```python
from build123d import *

# Parameters (mm, degrees)
F1_DEPTH = 3.175


with BuildPart() as f1:
    # F0 (on Front) → F1 (new body)
    with BuildSketch(Plane.XZ):
        Polygon((-109.02407, -38.0746), (-136.525, -38.0746), (-136.525, 0.0254), (-86.268388, 0.0254), (-38.200188, 0.0254), (136.525, 0.0254), (136.525, -38.0746), (0, -38.0746), (-16.379747, -38.0746), (-17.745636, -41.2496), (139.7, -41.2496), (139.7, 0.0254), (177.8, 0.0254), (177.8, 3.229479), (117.504079, 63.5254), (-117.504079, 63.5254), (-177.829079, 3.2004), (-177.8, 0.0254), (-139.7, 0.0254), (-139.7, -41.2496), (-61.467241, -41.2496), (-63.375022, -38.0746), (-86.524069, -38.0746), align=None)
        Polygon((-141.752446, 3.415089), (-173.407102, 3.132249), (-152.280724, 24.258627), (-116.353083, 60.186267), (-115.853459, 60.18446), (-76.571651, 60.042381), (-33.768375, 59.887564), (117.197821, 59.34153), (170.335695, 6.203656), (0, 4.681674), (-33.768375, 4.379947), (-51.768549, 4.219112), (-51.998988, 3.506442), (-52.306652, 4.214304), (-92.559852, 3.854634), (-131.528538, 3.506442), (-138.940506, 3.440214), align=None, mode=Mode.SUBTRACT)
    extrude(amount=F1_DEPTH)


solid = f1.part
```
Can you work these out from the model? Positions are in its coordinate system, mm. Give positions to 0.01 mm unless a question says otherwise; leave off trailing zeros. Write each loop counter-clockwise with the first axis right and the second up, starting at its lowest first coordinate (ties: lowest second). Pieces come first, ordered by that corner, then holes. Notation, with made-up numbers: (-16.5, -40) -> (14.5, -40) arc R3 cw to (14.5, -35) -> close; hole circle Ø9 at (-15, 83). An arc over 180 degrees is marked (long way). Write item = value, one per line.
(1) Thinking about a two-plate mould opening in X: for faces 1 (the face through (12, 0, 4)), 2 (the face through (143.395, -1.565, 33.145)), 3 (the face through (-147.24, -1.57, 33.79)), 4 (the face through (148.07, -1.57, 32.96)), which applies, released by +X, released by -X, zero draft, split by the parting line, or undercut?
Worked out:
face_1 = zero draft
face_2 = undercut
face_3 = released by -X
face_4 = released by +X
(2) Suppose I cut it at B-B on x = 4.5. Write out the boundary of the cut face in (y, z) (3 decimals).
Worked out:
outline = (-3.175, -41.25) -> (0, -41.25) -> (0, -38.075) -> (-3.175, -38.075) -> close; (-3.175, 0.025) -> (0, 0.025) -> (0, 4.722) -> (-3.175, 4.722) -> close; (-3.175, 59.749) -> (0, 59.749) -> (0, 63.525) -> (-3.175, 63.525) -> close
(3) Suppose I cut it at D-D on x = 81.5. Write out the boundary of the cut face in (y, z) (3 decimals), then the cut area to 3 significant figures.
Worked out:
outline = (-3.175, -41.25) -> (0, -41.25) -> (0, -38.075) -> (-3.175, -38.075) -> close; (-3.175, 0.025) -> (0, 0.025) -> (0, 5.41) -> (-3.175, 5.41) -> close; (-3.175, 59.471) -> (0, 59.471) -> (0, 63.525) -> (-3.175, 63.525) -> close
area = 40.1 mm^2
(4) Suppose I cut it at C-C on x = -56.5. Write out the boundary of the cut face in (y, z) (3 decimals).
Worked out:
outline = (-3.175, 0.025) -> (0, 0.025) -> (0, 4.177) -> (-3.175, 4.177) -> close; (-3.175, 59.97) -> (0, 59.97) -> (0, 63.525) -> (-3.175, 63.525) -> close
(5) I need wall thicknesses on probe 1 along Z at (x, y) = (-92.5, -1.3); probe 2 along X at (y, z) = (-1.3, -26.5) (3 decimals); probe 3 along Z at (x, y) = (39.5, -2.4). Which ranges of each line are inside material? Lowest first, please. Write a range as from..to.
Worked out:
probe_1 = -41.25..-38.07, 0.03..3.86, 60.1..63.53
probe_2 = -139.7..-136.525, 136.525..139.7
probe_3 = -41.25..-38.07, 0.03..5.03, 59.62..63.53
(6) Suppose I cut it at A-A on z = 52. Write out the boundary of the cut face in (x, y) (3 decimals).
Worked out:
outline = (-129.029, -3.175) -> (-124.539, -3.175) -> (-124.539, 0) -> (-129.029, 0) -> close; (124.539, -3.175) -> (129.029, -3.175) -> (129.029, 0) -> (124.539, 0) -> close
(7) I'm going to push flat-ended pins straight in: P1, Ø1.6, axis at x = -153, y = -1, coming from the -Z side; P2, Ø1, axis at y = -1.5, z = -20.5, coming from the +X side; P3, Ø10, axis at x = 114.5, z = 52, coming from the -Y side; P4, Ø1, axis at y = -1.5, z = -11, coming from the -X side. Where does each tip first touch, or does it pass through?
Worked out:
P1 = 0.03
P2 = 139.7
P3 = through
P4 = -139.7
